from build123d import *

# Parameters (mm, degrees)
PAD_DEPTH       = 5
POCKET_DEPTH    = 5.001
SKETCH002_W     = 10
SKETCH002_H     = 5
POCKET001_DEPTH = 2.5


with BuildPart() as part:
    # Sketch → Pad (new body)
    with BuildSketch(Plane.XY):
        Polygon((-12.374988, 34), (0, 0), (41.917536, 0), (28.180149, 5), (8.180149, 5), (-2.374988, 34), align=None)
    extrude(amount=PAD_DEPTH)

    # Sketch001 (on Face8 of Pad) → Pocket (cut, through all)
    with BuildSketch(Plane.XY.offset(5)):
        with BuildLine():
            ThreePointArc((-6.874988, 30.8), (-8.674988, 29), (-6.874988, 27.2))
            Line((-6.874988, 27.2), (-3.874988, 27.2))
            ThreePointArc((-3.874988, 27.2), (-2.074988, 29), (-3.874988, 30.8))
            Line((-3.874988, 30.8), (-6.874988, 30.8))
        make_face()
        with BuildLine():
            ThreePointArc((-3.374988, 20.8), (-5.174988, 19), (-3.374988, 17.2))
            Line((-3.374988, 17.2), (-0.374988, 17.2))
            ThreePointArc((-0.374988, 17.2), (1.425012, 19), (-0.374988, 20.8))
            Line((-0.374988, 20.8), (-3.374988, 20.8))
        make_face()
        with BuildLine():
            ThreePointArc((0.125012, 10.8), (-1.674988, 9), (0.125012, 7.2))
            Line((0.125012, 7.2), (3.125012, 7.2))
            ThreePointArc((3.125012, 7.2), (4.925012, 9), (3.125012, 10.8))
            Line((3.125012, 10.8), (0.125012, 10.8))
        make_face()
    extrude(amount=-POCKET_DEPTH, mode=Mode.SUBTRACT)

    # Sketch002 (on Face8 of Pocket) → Pocket001 (cut)
    with BuildSketch(Plane(origin=(0, 5, 0), x_dir=(-1, 0, 0), z_dir=(0, 1, 0))):
        with Locations((-18.180149, 2.5)):
            Rectangle(SKETCH002_W, SKETCH002_H)
    extrude(amount=-POCKET001_DEPTH, mode=Mode.SUBTRACT)


solid = part.part
The model under review builds one solid part; all positions refer to its coordinate system, in mm. A direction names the side the tool comes from. Coordinates: 2 decimals unless noted, no trailing zeros. Loops run counter-clockwise (first coordinate to the right, second up) from the corner with the lowest first, then second, coordinate; pieces in that order, holes last. Notation, with made-up numbers: M 85.5,63.5 L 116.5,63.5 A9 cw 116.5,79.5 Z; hole C -21,-31 d2. An arc over 180 degrees is marked long. Put each result on its own line as item: value. Start each with the question number.
Q1. Add section D-D (y = 15.5). Write out the cut boundary in (x, z).
Q2. Clearance check with flat-ended pins moving along their axes: pin 1 (2 mm diameter, centred on y = 18.5, z = 4, fed in from +X); pin 2 (0.8 mm diameter, centred on y = 3, z = 3, fed in from -X); pin 3 (3 mm diameter, centred on x = 34, z = 4.5, fed in from +Y). State where each tip first meets the part, or that it passes through.
Q3. The part is to be moulded in two halves that separate along X. For faces 1 (the flat face through (-6.274, 17.238, 2.465)), 2 (the flat face through (-5, 27.2, 3)), 3 (the cylindrical face through (-1.675, 9.04, 2.535)), 4 (the flat face through (5, 13, 0)), say which applies: +X half, -X half, draft (parallel to the pull), parting line (faces both ways), or undercut.
Q4. Add section B-B (y = 19). Write out the cut boundary in (x, z).
Q5. For faces 5 (the flat face through (23.18, 4, 2)), 6 (the flat face through (5, 13, 5)), 7 (the cylindrical face through (1.425, 18.96, 2.535)), list the 3-axis set-ups (+Z, -Z, +X, -X, +Y, -Y) from which the entire face can be reached by the end or side of a thin tool; tool diameter is ignored.
Q6. Wall thickness on line 1 (Y direction, x = 9, z = 0.45); line 2 (Y direction, x = 18.5, z = 3.2); line 3 (X direction, y = 20.5, z = 3.65): over which ranges is each line inside the solid? List them lowest first.
Q7. Add section C-C (x = 12). Write out the cut boundary in (y, z).
Q8. Add section A-A (z = 0.9). Write out the cut boundary in (x, y), and give its area (3 significant figures).
Answers:
1. outline: M -5.64,0 L 4.36,0 L 4.36,5 L -5.64,5 Z
2. pin 1: stops at x = 3.63
2. pin 2: stops at x = -1.24
2. pin 3: stops at y = 3.43
3. face 1: -X half
3. face 2: undercut
3. face 3: undercut
3. face 4: draft
4. outline: M -6.92,0 L -5.17,0 L -5.17,5 L -6.92,5 Z; M 1.43,0 L 3.08,0 L 3.08,5 L 1.43,5 Z
5. face 5: +Z, -Z, +Y
5. face 6: +Z, +X, -X, +Y, -Y
5. face 7: +Z, -Z
6. line 1: y = 0 to 5
6. line 2: y = 0 to 2.5
6. line 3: x = -7.46 to -4.37, 0.62 to 2.54
7. outline: M 0,0 L 5,0 L 5,5 L 0,5 Z
8. outline: M -12.37,34 L 0,0 L 41.92,0 L 28.18,5 L 23.18,5 L 23.18,2.5 L 13.18,2.5 L 13.18,5 L 8.18,5 L -2.37,34 Z; hole M -6.87,27.2 L -3.87,27.2 A1.8 ccw -3.87,30.8 L -6.87,30.8 A1.8 ccw Z; hole M -3.37,17.2 L -0.37,17.2 A1.8 ccw -0.37,20.8 L -3.37,20.8 A1.8 ccw Z; hole M 0.13,7.2 L 3.13,7.2 A1.8 ccw 3.13,10.8 L 0.13,10.8 A1.8 ccw Z
8. area: 382 mm^2
